from build123d import *

# Parameters (mm, degrees)
F0_W     = 101.6
F0_H     = 50.8
F1_DEPTH = 101.6


with BuildPart() as f1:
    # F0 (on Front) → F1 (new body)
    with BuildSketch(Plane.XZ):
        Polygon((52.296527, 96.696837), (-74.703473, 96.696837), (-74.703473, -55.703163), (52.296527, -55.703163), (52.296527, -4.903163), align=None)
        Polygon((153.896527, -4.903163), (52.296527, 96.696837), (52.296527, -4.903163), align=None)
        with Locations((103.096527, -30.303163)):
            Rectangle(F0_W, F0_H)
    extrude(amount=F1_DEPTH)


solid = f1.part
Could you check a few things on this model? Use its own coordinates, in mm. Coordinates: 2 decimals unless noted, no trailing zeros. Order: outer loops, then holes, each group sorted by start corner. A loop starts at its lowest first (then second) coordinate and runs counter-clockwise, first axis right, second up. Notation, with made-up numbers: (84, -5) - (110, -5) arc R30 cw to (110, 32) - close; hole circle Ø1 at (-30.5, 52). An arc over 180 degrees is marked (long way). Answer in a Markdown table with one row per item. Add a question column.
(1) If we section it at A-A, the plane y = -95: Please give me the cut outline in (x, z).
(2) Will this pin go through, and if not, where does the flat tip stop? pin 1 (4 mm diameter, centred on y = -54.5, z = 59.5, fed in from +X).
(3) If we section it at B-B, the plane x = 106: Please give me the cut outline in (y, z).
(4) If we section it at C-C, the plane z = 24: Please give me the cut outline in (x, y), then the cut area to 3 significant figures.
(5) I need wall thicknesses on L1, parallel to Z at x = 109.5, y = -86; L2, parallel to Z at x = 79, y = -96; L3, parallel to X at y = -38, z = 75. Which ranges of each line are inside material? Lowest first, please.
Results are:
| question | item | result |
|---|---|---|
| 1 | outline | (-74.7, -55.7) - (153.9, -55.7) - (153.9, -4.9) - (52.3, 96.7) - (-74.7, 96.7) - close |
| 2 | pin 1 | stops at x = 91.49 |
| 3 | outline | (-101.6, -55.7) - (0, -55.7) - (0, 42.99) - (-101.6, 42.99) - close |
| 4 | outline | (-74.7, -101.6) - (124.99, -101.6) - (124.99, 0) - (-74.7, 0) - close |
| 4 | area | 20,300 mm2 |
| 5 | L1 | z = -55.7 to 39.49 |
| 5 | L2 | z = -55.7 to 69.99 |
| 5 | L3 | x = -74.7 to 73.99 |
